Design review of the part built by this model. Coordinates are the model's own, in mm. Face numbers are marked on the shaded views. A direction names the side the tool comes from. Coordinates: 2 decimals unless noted, no trailing zeros. Write each loop counter-clockwise with the first axis right and the second up, starting at its lowest first coordinate (ties: lowest second). Pieces come first, ordered by that corner, then holes. Notation, with made-up numbers: (30, 38.5) -> (72, 38.5) arc R18 cw to (72, 58.5) -> close; hole circle Ø4 at (79, 41.25). An arc over 180 degrees is marked (long way). Write item = value, one per line. Start each with the question number.
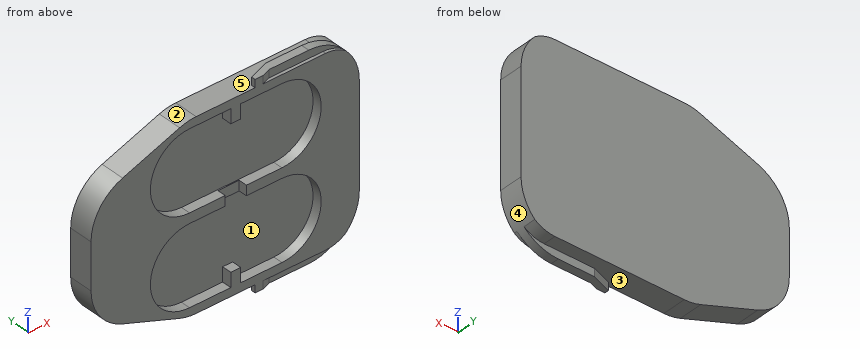
```python
from build123d import *

# Parameters (mm, degrees)
EXTRUDE_1_DEPTH     = 8.5
CUT_EXTRUDE_1_DEPTH = 3.4
SKETCH_7_W          = 3.5
SKETCH_7_H          = 5.05
EXTRUDE_2_DEPTH     = 3.4
SKETCH_8_W          = 7.5
SKETCH_8_H          = 3.5
CUT_EXTRUDE_2_DEPTH = 3
EXTRUDE_3_DEPTH     = 2.75
FILLET_2_R          = 12
FILLET_3_R          = 17
FILLET_4_R          = 17


with BuildPart() as part:
    # 草图1 → 凸台-拉伸1 (new body)
    with BuildSketch(Plane(origin=(0, 0, 0), x_dir=(1, 0, 0), z_dir=(0, 1, 0))):
        Polygon((-47.5, 20), (-13.3, 32.5), (47.5, 32.5), (47.5, -32.5), (-13.3, -32.5), (-47.5, -20), align=None)
    extrude(amount=EXTRUDE_1_DEPTH)

    # 草图3 → 切除-拉伸1 (cut)
    with BuildSketch(Plane.XZ):
        with BuildLine():
            Line((-12.6, 29.55), (20.1, 29.55))
            ThreePointArc((20.1, 29.55), (34, 15.65), (20.1, 1.75))
            Line((20.1, 1.75), (-12.6, 1.75))
            ThreePointArc((-12.6, 1.75), (-26.5, 15.65), (-12.6, 29.55))
        make_face()
        with BuildLine():
            Line((-12.6, -29.55), (20.1, -29.55))
            ThreePointArc((20.1, -29.55), (34, -15.65), (20.1, -1.75))
            Line((20.1, -1.75), (-12.6, -1.75))
            ThreePointArc((-12.6, -1.75), (-26.5, -15.65), (-12.6, -29.55))
        make_face()
    extrude(amount=-CUT_EXTRUDE_1_DEPTH, mode=Mode.SUBTRACT)

    # 草图7 → 凸台-拉伸2 (add)
    with BuildSketch(Plane.XZ.offset(-3.4)):
        with Locations((3.75, 27.025)):
            Rectangle(SKETCH_7_W, SKETCH_7_H)
    extrude_2 = extrude(amount=EXTRUDE_2_DEPTH)

    # 镜向1: 凸台-拉伸2 across plane
    add(extrude_2.mirror(Plane.XY))

    # 草图8 → 切除-拉伸2 (cut)
    with BuildSketch(Plane.XZ):
        with Locations((3.75, 0)):
            Rectangle(SKETCH_8_W, SKETCH_8_H)
    extrude(amount=-CUT_EXTRUDE_2_DEPTH, mode=Mode.SUBTRACT)

    # 草图10 → 凸台-拉伸3 (add)
    with BuildSketch(Plane.XY.offset(32.5)):
        Polygon((16.429732781, 1.1), (47.5, 1.1), (47.5, 4), (17.642356602, 4), (10.6, 1.44163271), (10.6, 0), (13.401789026, 0), align=None)
    extrude_3 = extrude(amount=EXTRUDE_3_DEPTH)

    # 镜向2: 凸台-拉伸3 across plane
    add(extrude_3.mirror(Plane.XY))

    # 圆角2
    fillet_2_edges = [part.edges().sort_by_distance(p)[0] for p in [
        (47.5, 6.25, 32.5),
        (47.5, 0.55, -32.5),
        (47.5, 6.25, -32.5),
        (47.5, 0.55, 32.5),
    ]]
    fillet(fillet_2_edges, radius=FILLET_2_R)

    # 圆角3
    fillet_3_edges = [part.edges().sort_by_distance(p)[0] for p in [
        (47.5, 2.55, 35.25),
        (47.5, 2.55, -35.25),
    ]]
    fillet(fillet_3_edges, radius=FILLET_3_R)

    # 圆角4
    fillet_4_edges = [part.edges().sort_by_distance(p)[0] for p in [
        (-13.3, 4.25, 32.5),
        (-47.5, 4.25, 20),
        (-47.5, 4.25, -20),
        (-13.3, 4.25, -32.5),
    ]]
    fillet(fillet_4_edges, radius=FILLET_4_R)


solid = part.part
```
(1) For the marked faces 4 and 5, list the 3-axis set-ups (+Z, -Z, +X, -X, +Y, -Y) from which the entire face can be reached by the end or side of a thin tool; tool diameter is ignored.
(2) Mouldability with a two-part tool opening along X and no side actions: class the marked faces 1, 2 and 3 as pulls with the +X half, pulls with the -X half, needs draft (parallel to the pull), parting line crosses it, or undercut.
(3) For pin 1 Ø3.5 at (y, z) = (2, -27.5) entering from +X; pin 2 Ø2.5 at (x, y) = (8, 1.5) entering from +Z; pin 3 Ø1.6 at (y, z) = (1, -34) entering from -X, all flat-tipped, find the tip position at first contact; note any pin that passes through.
(4) For line 1 (Z direction, x = 17.5, y = 2.25); line 2 (Z direction, x = -2.5, y = 1.5); line 3 (Y direction, x = 20, z = -16), list the stretches that pass through material, from the lowest coordinate up.
(5) Take a section at A-A, the plane z = -17. State the section outline as (x, y) points, then the cut area to 3 significant figures.
(6) Take a section at B-B, the plane x = -8.5. State the section outline as (y, z) points.
(7) Take a section at D-D, the plane x = 26. State the section outline as (y, z) points.
(8) Take a section at C-C, the plane y = 5.25. State the section outline as (x, z) points.
Report:
q1.face_4 = -Z, +X, +Y, -Y
q1.face_5 = +Z, -X, +Y
q2.face_1 = undercut
q2.face_2 = pulls with the -X half
q2.face_3 = needs draft
q3.pin_1 = 45.76
q3.pin_2 = 32.5
q3.pin_3 = 10.6
q4.line_1 = -35.25 to -29.55, -1.75 to 1.75, 29.55 to 35.25
q4.line_2 = -32.5 to -29.55, -1.75 to 1.75, 29.55 to 32.5
q4.line_3 = 3.4 to 8.5
q5.outline = (-44.99, 0) -> (-26.43, 0) -> (-26.43, 3.4) -> (33.93, 3.4) -> (33.93, 0) -> (47.5, 0) -> (47.5, 8.5) -> (-44.99, 8.5) -> close
q5.area = 581 mm2
q6.outline = (0, -32.5) -> (8.5, -32.5) -> (8.5, 32.5) -> (0, 32.5) -> (0, 29.55) -> (3.4, 29.55) -> (3.4, 1.75) -> (0, 1.75) -> (0, -1.75) -> (3.4, -1.75) -> (3.4, -29.55) -> (0, -29.55) -> close
q7.outline = (0, -32.5) -> (1.1, -32.5) -> (1.1, -35.25) -> (4, -35.25) -> (4, -32.5) -> (8.5, -32.5) -> (8.5, 32.5) -> (4, 32.5) -> (4, 35.25) -> (1.1, 35.25) -> (1.1, 32.5) -> (0, 32.5) -> (0, 28.24) -> (3.4, 28.24) -> (3.4, 3.06) -> (0, 3.06) -> (0, -3.06) -> (3.4, -3.06) -> (3.4, -28.24) -> (0, -28.24) -> close
q8.outline = (-47.5, -8.11) arc R17 ccw to (-36.34, -24.08) -> (-16.13, -31.47) arc R17 ccw to (-10.29, -32.5) -> (35.5, -32.5) arc R12 ccw to (42.66, -30.13) arc R17 ccw to (47.5, -18.25) -> (47.5, 18.25) arc R17 ccw to (42.66, 30.13) arc R12 ccw to (35.5, 32.5) -> (-10.29, 32.5) arc R17 ccw to (-16.13, 31.47) -> (-36.34, 24.08) arc R17 ccw to (-47.5, 8.11) -> close
